Source: CAD feature listing. Evaluate the final solid. Frame: model axes, mm. Give positions to 0.01 mm unless a question says otherwise; leave off trailing zeros. Order: outer loops, then holes, each group sorted by start corner. A loop starts at its lowest first (then second) coordinate and runs counter-clockwise, first axis right, second up. Notation, with made-up numbers: M 76.25,-29 L 97.25,-29 A29 ccw 97.25,8 Z; hole C -5.75,-31.5 d5. An arc over 180 degrees is marked long. Answer in a Markdown table with one row per item. Add a question column.
(1) Section query B-B, the plane y = -7. Return loops of the section in (x, z).
(2) Section query D-D, the plane y = 3. Return loops of the section in (x, z), plus the area to 3 significant figures.
(3) Material intervals for line 1 along Y through (x, z) = (-17, 3.75); line 2 along Y through (x, z) = (-6, 4.5); line 3 along X through (y, z) = (3.75, 1.75), sorted ascending.
(4) Section query A-A, the plane x = 17. Return loops of the section in (y, z), plus the area to 3 significant figures.
(5) Section query C-C, the plane z = 4. Return loops of the section in (x, y), plus the area to 3 significant figures.
from build123d import *

# Parameters (mm, degrees)
F0_W     = 50
F0_H     = 26
F1_DEPTH = 6.35
F2_R     = 1.1303
F3_DEPTH = 6.351
F5_DEPTH = 6.351
F6_R     = 1
F7_R     = 3
F8_R     = 1


with BuildPart() as f1:
    # F0 (on Top) → F1 (new body)
    with BuildSketch(Plane.XY):
        Rectangle(F0_W, F0_H)
    extrude(amount=F1_DEPTH)

    # F2 (on face) → F3 (cut, through all)
    with BuildSketch(Plane.XY.offset(6.35)):
        with Locations((-17, 10)):
            Circle(F2_R)
        with Locations((-17, 3)):
            Circle(F2_R)
        with Locations((17, 3)):
            Circle(F2_R)
        with Locations((17, 10)):
            Circle(F2_R)
    extrude(amount=-F3_DEPTH, mode=Mode.SUBTRACT)

    # F4 (on face) → F5 (cut, through all)
    with BuildSketch(Plane.XY.offset(6.35)):
        with BuildLine():
            Line((12.5, -5), (-12.5, -5))
            ThreePointArc((-12.5, -5), (-14.5, -7), (-12.5, -9))
            Line((-12.5, -9), (12.5, -9))
            ThreePointArc((12.5, -9), (14.5, -7), (12.5, -5))
        make_face()
    extrude(amount=-F5_DEPTH, mode=Mode.SUBTRACT)

    # F6
    f6_edges = [f1.edges().sort_by_distance(p)[0] for p in [
        (-25, 13, 3.175),
        (25, 13, 3.175),
        (0, -5, 6.35),
        (0, -5, 0),
    ]]
    fillet(f6_edges, radius=F6_R)

    # F7
    f7_edges = [f1.edges().sort_by_distance(p)[0] for p in [
        (-25, -13, 3.175),
        (25, -13, 3.175),
    ]]
    fillet(f7_edges, radius=F7_R)

    # F8
    f8_edges = [f1.edges().sort_by_distance(p)[0] for p in [
        (-25, 1, 6.35),
        (-25, 1, 0),
    ]]
    fillet(f8_edges, radius=F8_R)


solid = f1.part
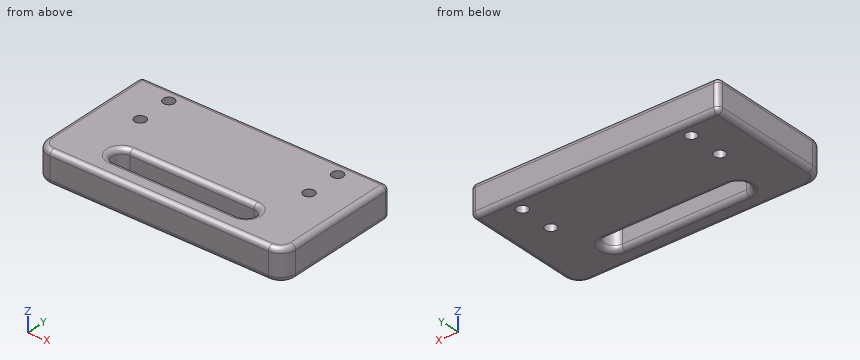
Values follow:
| question | item | result |
|---|---|---|
| 1 | outline | M -25,1 A1 ccw -24,0 L -15.5,0 A1 ccw -14.5,1 L -14.5,5.35 A1 ccw -15.5,6.35 L -24,6.35 A1 ccw -25,5.35 Z; M 14.5,1 A1 ccw 15.5,0 L 24,0 A1 ccw 25,1 L 25,5.35 A1 ccw 24,6.35 L 15.5,6.35 A1 ccw 14.5,5.35 Z |
| 2 | outline | M -25,1 A1 ccw -24,0 L -18.13,0 L -18.13,6.35 L -24,6.35 A1 ccw -25,5.35 Z; M -15.87,0 L 15.87,0 L 15.87,6.35 L -15.87,6.35 Z; M 18.13,0 L 24,0 A1 ccw 25,1 L 25,5.35 A1 ccw 24,6.35 L 18.13,6.35 Z |
| 2 | area | 288 mm² |
| 3 | line 1 | y = -13 to 1.87, 4.13 to 8.87, 11.13 to 13 |
| 3 | line 2 | y = -13 to -9, -5 to 13 |
| 3 | line 3 | x = -25 to -17.85, -16.15 to 16.15, 17.85 to 25 |
| 4 | outline | M -13,1 A1 ccw -12,0 L 1.87,0 L 1.87,6.35 L -12,6.35 A1 ccw -13,5.35 Z; M 4.13,0 L 8.87,0 L 8.87,6.35 L 4.13,6.35 Z; M 11.13,0 L 12,0 A1 ccw 13,1 L 13,5.35 A1 ccw 12,6.35 L 11.13,6.35 Z |
| 4 | area | 136 mm² |
| 5 | outline | M -25,-10 A3 ccw -22,-13 L 22,-13 A3 ccw 25,-10 L 25,12 A1 ccw 24,13 L -24,13 A1 ccw -25,12 Z; hole C -17,3 d2.26; hole C -17,10 d2.26; hole M -12.5,-9 L 12.5,-9 A2 ccw 12.5,-5 L -12.5,-5 A2 ccw Z; hole C 17,3 d2.26; hole C 17,10 d2.26 |
| 5 | area | 1,170 mm² |
